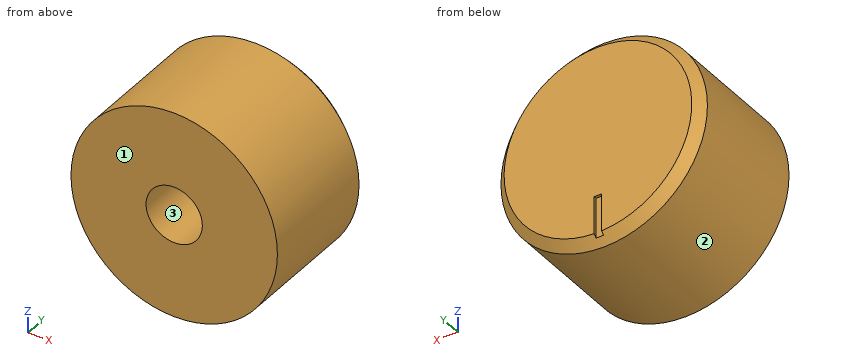
from build123d import *

# Parameters (mm, degrees)
SKETCH1_R           = 11
BOSS_EXTRUDE1_DEPTH = 14
CHAMFER1_SIZE       = 1
SKETCH3_W           = 0.8
SKETCH3_H           = 5
CUT_EXTRUDE1_DEPTH  = 0.3
SKETCH4_R           = 3
CUT_EXTRUDE2_DEPTH  = 10


with BuildPart() as part:
    # Sketch1 → Boss-Extrude1 (new body)
    with BuildSketch(Plane(origin=(0, 0, 0), x_dir=(1, 0, 0), z_dir=(0, 1, 0))):
        with Locations(Location((0, 0, 0), (0, 0, 270))):
            Circle(SKETCH1_R)
    extrude(amount=BOSS_EXTRUDE1_DEPTH)

    # Chamfer1
    chamfer1_edges = [part.edges().sort_by_distance(p)[0] for p in [
        (0, 14, -11),
    ]]
    chamfer(chamfer1_edges, length=CHAMFER1_SIZE)

    # Sketch3 → Cut-Extrude1 (cut)
    with BuildSketch(Plane(origin=(0, 14, 0), x_dir=(1, 0, 0), z_dir=(0, 1, 0))):
        with Locations((0, 8.5)):
            Rectangle(SKETCH3_W, SKETCH3_H)
    extrude(amount=-CUT_EXTRUDE1_DEPTH, mode=Mode.SUBTRACT)

    # Sketch4 → Cut-Extrude2 (cut)
    with BuildSketch(Plane.XZ):
        with Locations(Location((0, 0, 0), (0, 0, 270))):
            Circle(SKETCH4_R)
    extrude(amount=-CUT_EXTRUDE2_DEPTH, mode=Mode.SUBTRACT)


solid = part.part
Geometry: final body of the model. Coordinates: model frame, mm. Face numbers are marked on the shaded views. Round coordinates to 2 decimals unless told otherwise and drop trailing zeros. Order: outer loops, then holes, each group sorted by start corner. A loop starts at its lowest first (then second) coordinate and runs counter-clockwise, first axis right, second up.
Q1. Section A-A, the plane x = 0. Output: boundary loops of the cut face in (y, z), and give its area (3 significant figures).
Result sheet:
outline: (0, -11) - (13, -11) - (13.7, -10.3) - (13.7, -6) - (14, -6) - (14, 10) - (13, 11) - (0, 11) - (0, 3) - (10, 3) - (10, -3) - (0, -3) - close
area: 246 mm2
Q2. Section C-C, the plane y = 1. Output: boundary loops of the cut face in (x, z), and give its area (3 significant figures).
Result sheet:
outline: circle Ø22 at (0, 0); hole circle Ø6 at (0, 0)
area: 352 mm2
Q3. Mould query, pull axis Z, two halves, no side actions, for the marked faces 1, 2 and 3. Classes: released by +Z, released by -Z, zero draft, split by the parting line, or undercut.
Result sheet:
face 1: zero draft
face 2: split by the parting line
face 3: undercut
Q4. Section B-B, the plane z = 0. Output: boundary loops of the cut face in (x, y), and give its area (3 significant figures).
Result sheet:
outline: (-11, 0) - (-3, 0) - (-3, 10) - (3, 10) - (3, 0) - (11, 0) - (11, 13) - (10, 14) - (-10, 14) - (-11, 13) - close
area: 247 mm2
Q5. Pin query (flat end, axial travel): pin 1 (8 mm diameter, centred on y = 12.5, z = 6, fed in from -X); pin 2 (8 mm diameter, centred on y = 5.5, z = 8.5, fed in from +X); pin 3 (2 mm diameter, centred on x = 5, y = 11, fed in from +Z); pin 4 (4 mm diameter, centred on x = 6, z = -1, fed in from -Y). Return the tip coordinate at first contact, or that it passes through.
Result sheet:
pin 1: stops at x = -10.82
pin 2: stops at x = 10.04
pin 3: stops at z = 10.25
pin 4: stops at y = 0
Q6. Material intervals for probe 1 along X at (y, z) = (4.25, 0); probe 2 along Y at (x, z) = (-0.5, 0); probe 3 along X at (y, z) = (3.75, -1.5), sorted ascending.
Result sheet:
probe 1: x = -11 to -3, 3 to 11
probe 2: y = 10 to 14
probe 3: x = -10.9 to -2.6, 2.6 to 10.9
